from build123d import *

# Parameters (mm, degrees)
SKETCH1_W           = 150
SKETCH1_H           = 150
BOSS_EXTRUDE1_DEPTH = 10
SKETCH2_R           = 4
SKETCH2_R_2         = 2
CUT_EXTRUDE1_DEPTH  = 10


with BuildPart() as part:
    # Sketch1 → Boss-Extrude1 (new body)
    with BuildSketch(Plane(origin=(0, 0, 0), x_dir=(1, 0, 0), z_dir=(0, 1, 0))):
        Rectangle(SKETCH1_W, SKETCH1_H)
    extrude(amount=BOSS_EXTRUDE1_DEPTH)

    # Sketch2 → Cut-Extrude1 (cut)
    with BuildSketch(Plane(origin=(0, 10, 0), x_dir=(1, 0, 0), z_dir=(0, 1, 0))):
        with Locations((23, 5)):
            Circle(SKETCH2_R)
        with Locations((-23, 5)):
            Circle(SKETCH2_R)
        with Locations((-65, 13)):
            Circle(SKETCH2_R_2)
        with Locations((-39, 13)):
            Circle(SKETCH2_R_2)
        with Locations((-65, -13)):
            Circle(SKETCH2_R_2)
        with Locations((-39, -13)):
            Circle(SKETCH2_R_2)
        with Locations((39, 13)):
            Circle(SKETCH2_R_2)
        with Locations((65, 13)):
            Circle(SKETCH2_R_2)
        with Locations((65, -13)):
            Circle(SKETCH2_R_2)
        with Locations((39, -13)):
            Circle(SKETCH2_R_2)
    extrude(amount=-CUT_EXTRUDE1_DEPTH, mode=Mode.SUBTRACT)


solid = part.part
CAD build for the part. Positions are in the model's coordinates, mm. Coordinates: 2 decimals unless noted, no trailing zeros. Write each loop counter-clockwise with the first axis right and the second up, starting at its lowest first coordinate (ties: lowest second). Pieces come first, ordered by that corner, then holes. Notation, with made-up numbers: (-19, -0.75) - (7, -0.75) arc R19 ccw to (7, 14.25) - close; hole circle Ø7 at (36, -16). An arc over 180 degrees is marked (long way). Use a Markdown table: item, result. Add a question column.
Item 1: Band-saw the part on A-A, the plane z = 13. Give the cut face in (x, y).
Item 2: Mould opens along X. For faces 1 (the face through (-75, 5, 1)), 2 (the face through (-1, 5, -75)), 3 (the face through (-40.474, 5.07, 11.648)) say: pulls with the +X half, pulls with the -X half, needs draft (parallel to the pull), parting line crosses it, or undercut.
Item 3: Band-saw the part on C-C, the plane x = 23. Give the cut face in (y, z).
Item 4: Drill centre lines: L1, parallel to Z at x = 39, y = 2.5; L2, parallel to X at y = 6.75, z = -13; L3, parallel to X at y = 3.75, z = -5. Where is each one in solid material? Low to high. Write a range as from..to.
Item 5: Band-saw the part on B-B, the plane x = -39. Give the cut face in (y, z), and give its area (3 significant figures).
Numbers:
| question | item | result |
|---|---|---|
| 1 | outline | (-75, 0) - (-67, 0) - (-67, 10) - (-75, 10) - close; (-63, 0) - (-41, 0) - (-41, 10) - (-63, 10) - close; (-37, 0) - (37, 0) - (37, 10) - (-37, 10) - close; (41, 0) - (63, 0) - (63, 10) - (41, 10) - close; (67, 0) - (75, 0) - (75, 10) - (67, 10) - close |
| 2 | face 1 | pulls with the -X half |
| 2 | face 2 | needs draft |
| 2 | face 3 | undercut |
| 3 | outline | (0, -75) - (10, -75) - (10, -9) - (0, -9) - close; (0, -1) - (10, -1) - (10, 75) - (0, 75) - close |
| 4 | L1 | -75..-15, -11..11, 15..75 |
| 4 | L2 | -75..-67, -63..-41, -37..37, 41..63, 67..75 |
| 4 | L3 | -75..-27, -19..19, 27..75 |
| 5 | outline | (0, -75) - (10, -75) - (10, -15) - (0, -15) - close; (0, -11) - (10, -11) - (10, 11) - (0, 11) - close; (0, 15) - (10, 15) - (10, 75) - (0, 75) - close |
| 5 | area | 1,420 mm2 |
